Solid Edge part; units mm, degrees
sketch "Sketch1" plane through (0, 0, 0) normal (1, 0, 0) x (0, 1, 0)
  line L0 (0, 0) -> (-20, 0)
  line L1 (-20, 0) -> (-20, 3)
  line L2 (-20, 3) -> (-3, 3)
  line L3 (-3, 3) -> (-3, 20)
  line L4 (-3, 20) -> (0, 20)
  line L5 (0, 20) -> (0, 0)
extrude "Protrusion1" add sketch "Sketch1" along normal mid plane 200
sketch "Sketch2" plane through (0, 0, 0) normal (0, 0, 1) x (1, 0, 0)
  circle A0 centre (-65, -11.5) radius 3
  circle A1 centre (65, -11.5) radius 3
extrude "Cutout1" cut sketch "Sketch2" along normal up to next
sketch "Sketch3" plane through (0, 0, 0) normal (0, -1, 0) x (1, 0, 0)
  circle A0 centre (0, 11.5) radius 4
extrude "Cutout2" cut sketch "Sketch3" along normal up to next
Part model, mm, in its own coordinate system. A direction names the side the tool comes from. Coordinates: 2 decimals unless noted, no trailing zeros. Order: outer loops, then holes, each group sorted by start corner. A loop starts at its lowest first (then second) coordinate and runs counter-clockwise, first axis right, second up.
(1) Probe L1, parallel to X at y = -11.5, z = 0.75; L2, parallel to Z at x = 0, y = -2.1; L3, parallel to X at y = -1.6, z = 11.5. List the from-to ranges inside material, lowest first.
Check sheet entries:
L1: x = -100 to -68, -62 to 62, 68 to 100
L2: z = 0 to 7.5, 15.5 to 20
L3: x = -100 to -4, 4 to 100
(2) Pull direction Y, two halves, no side cores. Call faces 1 (the face through (-67.4, -9.7, 1.5)), 2 (the face through (-1, -10, 0)), 3 (the face through (-1, 0, 6)), 4 (the face through (62, -11.6, 1.5)): pulls with the +Y half, pulls with the -Y half, needs draft (parallel to the pull), parting line crosses it, or undercut.
Check sheet entries:
face 1: undercut
face 2: needs draft
face 3: pulls with the +Y half
face 4: undercut
(3) Slice it at D-D, the plane x = 65. Write the cut outline in (y, z).
Check sheet entries:
outline: (-20, 0) - (-14.5, 0) - (-14.5, 3) - (-20, 3) - close; (-8.5, 0) - (0, 0) - (0, 20) - (-3, 20) - (-3, 3) - (-8.5, 3) - close
(4) Slice it at C-C, the plane z = 11.5. Write the cut outline in (x, y).
Check sheet entries:
outline: (-100, -3) - (-4, -3) - (-4, 0) - (-100, 0) - close; (4, -3) - (100, -3) - (100, 0) - (4, 0) - close
(5) Slice it at B-B, the plane y = -11.5. Write the cut outline in (x, z).
Check sheet entries:
outline: (-100, 0) - (-68, 0) - (-68, 3) - (-100, 3) - close; (-62, 0) - (62, 0) - (62, 3) - (-62, 3) - close; (68, 0) - (100, 0) - (100, 3) - (68, 3) - close
(6) Slice it at A-A, the plane x = 0. Write the cut outline in (y, z), and give its area (3 significant figures).
Check sheet entries:
outline: (-20, 0) - (0, 0) - (0, 7.5) - (-3, 7.5) - (-3, 3) - (-20, 3) - close; (-3, 15.5) - (0, 15.5) - (0, 20) - (-3, 20) - close
area: 87.0 mm2
(7) Tool access for faces 5 (the face through (-1, -12, 3)), 6 (the face through (100, -6.3, 2.6)): list every direction of +Z, -Z, +X, -X, +Y, -Y with a clear straight run to the whole face (end or side of a thin tool).
Check sheet entries:
face 5: +Z, +X, -X, -Y
face 6: +Z, -Z, +X, +Y, -Y
(8) Pin check, flat tips, straight feed: pin 1 Ø3 at (x, y) = (46, -8.5) entering from -Z; pin 2 Ø8 at (x, y) = (-65, -11.5) entering from +Z; pin 3 Ø1 at (x, z) = (-3.5, 8.5) entering from -Y; pin 4 Ø3.5 at (x, y) = (65, -11.5) entering from +Z. Stop position of each tip, or through.
Check sheet entries:
pin 1: stops at z = 0
pin 2: stops at z = 3
pin 3: stops at y = -3
pin 4: passes through
